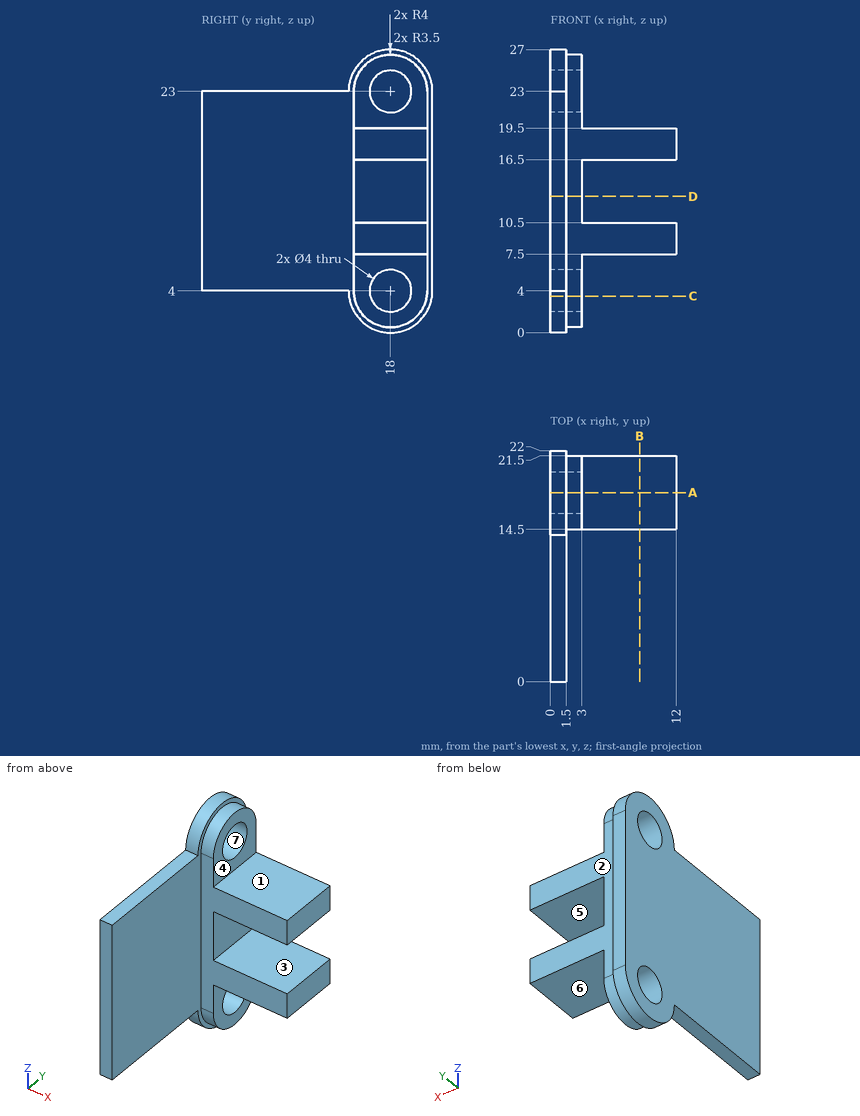
Drawing for the job (mm, zero at the part's lowest x, y, z). A direction names the side the tool comes from. Round coordinates to 2 decimals unless told otherwise and drop trailing zeros. Write each loop counter-clockwise with the first axis right and the second up, starting at its lowest first coordinate (ties: lowest second). Pieces come first, ordered by that corner, then holes. Notation, with made-up numbers: M 44.5,43 L 56.5,43 A31 cw 56.5,81 Z; hole C 68.25,19.25 d2. An arc over 180 degrees is marked long. Answer in a Markdown table with one row per item.
1. Saw through at C-C (z = 3.5). List the corners of the cut face in (x, y).
Geometry check:
| item | result |
|---|---|
| outline | M 0,14.03 L 1.5,14.03 L 1.5,14.54 L 3,14.54 L 3,16.06 L 0,16.06 Z; M 0,19.94 L 3,19.94 L 3,21.46 L 1.5,21.46 L 1.5,21.97 L 0,21.97 Z |
2. Probe L1, parallel to Z at x = 2.3, y = 18; L2, parallel to Z at x = 1.3, y = 18; L3, parallel to Z at x = 9.5, y = 20.75. List the from-to ranges inside material, lowest first. Write a range as [from, to].
Geometry check:
| item | result |
|---|---|
| L1 | [0.5, 2], [6, 21], [25, 26.5] |
| L2 | [0, 2], [6, 21], [25, 27] |
| L3 | [7.5, 10.5], [16.5, 19.5] |
3. Saw through at D-D (z = 13). List the corners of the cut face in (x, y).
Geometry check:
| item | result |
|---|---|
| outline | M 0,0 L 1.5,0 L 1.5,14.5 L 3,14.5 L 3,21.5 L 1.5,21.5 L 1.5,22 L 0,22 Z |
4. Mould opens along Z. For the marked faces 4, 5, 6 and 7 say: +Z half, -Z half, draft (parallel to the pull), parting line (faces both ways), or undercut.
Geometry check:
| item | result |
|---|---|
| face 4 | draft |
| face 5 | undercut |
| face 6 | -Z half |
| face 7 | undercut |
5. Which spindle directions (+Z, -Z, +X, -X, +Y, -Y) get a long thin tool onto all of the face, cutting with end or side? Do the marked faces 1, 2 and 3. Say none if no direction does.
Geometry check:
| item | result |
|---|---|
| face 1 | +Z, +X, +Y, -Y |
| face 2 | +Z, -Z, +X, +Y |
| face 3 | +X, +Y, -Y |
6. Saw through at B-B (x = 8.5). List the corners of the cut face in (y, z).
Geometry check:
| item | result |
|---|---|
| outline | M 14.5,7.5 L 21.5,7.5 L 21.5,10.5 L 14.5,10.5 Z; M 14.5,16.5 L 21.5,16.5 L 21.5,19.5 L 14.5,19.5 Z |
7. Flat gauge pins, fed straight in: P1, Ø3, axis at x = 10.5, y = 13.5, coming from the -Z side; P2, Ø5, axis at x = 6.5, z = 9.5, coming from the +Y side; P3, Ø4, axis at x = 3, y = 13, coming from the -Z side. Where does each tip first touch, or does it go through?
Geometry check:
| item | result |
|---|---|
| P1 | z = 7.5 |
| P2 | y = 21.5 |
| P3 | z = 2.2 |
8. Saw through at A-A (y = 18). List the corners of the cut face in (x, z).
Geometry check:
| item | result |
|---|---|
| outline | M 0,0 L 1.5,0 L 1.5,0.5 L 3,0.5 L 3,2 L 0,2 Z; M 0,6 L 3,6 L 3,7.5 L 12,7.5 L 12,10.5 L 3,10.5 L 3,16.5 L 12,16.5 L 12,19.5 L 3,19.5 L 3,21 L 0,21 Z; M 0,25 L 3,25 L 3,26.5 L 1.5,26.5 L 1.5,27 L 0,27 Z |
